Check sheet for the modelled part. Datum: model origin and axes. Units: mm. Face numbers are marked on the shaded views. A direction names the side the tool comes from. Give positions to 0.01 mm unless a question says otherwise; leave off trailing zeros. Loops run counter-clockwise (first coordinate to the right, second up) from the corner with the lowest first, then second, coordinate; pieces in that order, holes last. Notation, with made-up numbers: (41, 18.25) - (54, 18.25) arc R21 cw to (54, 40.25) - close; hole circle Ø5 at (38.5, -6). An arc over 180 degrees is marked (long way). Answer in a Markdown table with one row per item. Add a question column.
(1) Sectioned sample at B-B on z = 6. Enter the section's corners in (x, y).
(2) Sectioned sample at C-C on y = 1. Enter the section's corners in (x, z).
(3) Thickness scan on L1, parallel to Z at x = 53, y = 2; L2, parallel to Y at x = 39.5, z = 3.5. Record the ranges inside material, lowest first.
(4) Go/stop test with flat-tipped pins: P1, Ø6.5, axis at x = 59, z = 4.5, coming from the -Y side; P2, Ø1, axis at x = 37, y = 6.5, coming from the -Z side; P3, Ø9, axis at x = 21, z = 2, coming from the +Y side. Record where each tip stops, or that it passes through.
(5) Set-up check for the marked faces 1, 2 and 3: record each of +Z, -Z, +X, -X, +Y, -Y from which the full face is reachable in a straight line by a thin tool's end or side.
(6) Sectioned sample at A-A on x = 60.5. Enter the section's corners in (y, z).
from build123d import *

# Parameters (mm, degrees)
SKETCH1_W           = 80
SKETCH1_H           = 8.1
BOSS_EXTRUDE1_DEPTH = 20
CUT_EXTRUDE1_DEPTH  = 85


with BuildPart() as part:
    # Sketch1 → Boss-Extrude1 (new body)
    with BuildSketch(Plane.XY):
        with Locations((40, 4.05)):
            Rectangle(SKETCH1_W, SKETCH1_H)
    extrude(amount=BOSS_EXTRUDE1_DEPTH)

    # Sketch2 → Cut-Extrude1 (cut)
    with BuildSketch(Plane.ZY):
        Polygon((0, 8.1), (8, 8.1), (8, 5.9), (1.006469224, 5.9), (0, 5.9), align=None)
        Polygon((0, 0), (8, 0), (8, 2.2), (1.006469224, 2.2), (0, 2.2), align=None)
    extrude(amount=-CUT_EXTRUDE1_DEPTH, mode=Mode.SUBTRACT)


solid = part.part
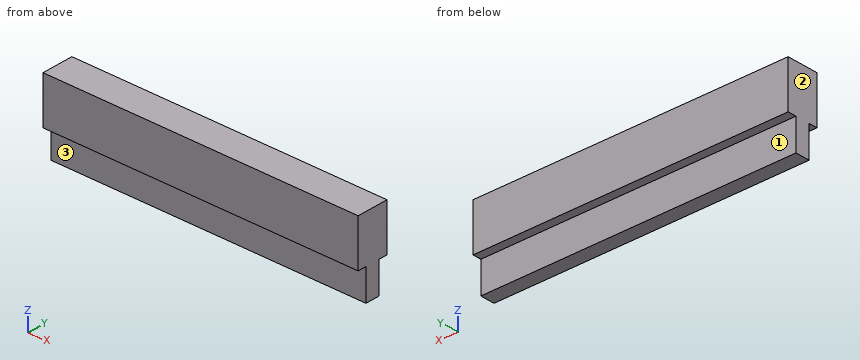
Reply:
| question | item | result |
|---|---|---|
| 1 | outline | (0, 2.2) - (80, 2.2) - (80, 5.9) - (0, 5.9) - close |
| 2 | outline | (0, 8) - (80, 8) - (80, 20) - (0, 20) - close |
| 3 | L1 | 8 to 20 |
| 3 | L2 | 2.2 to 5.9 |
| 4 | P1 | y = 2.2 |
| 4 | P2 | z = 8 |
| 4 | P3 | y = 5.9 |
| 5 | face 1 | -Z, +X, -X, +Y |
| 5 | face 2 | +Z, -Z, -X, +Y, -Y |
| 5 | face 3 | -Z, +X, -X, -Y |
| 6 | outline | (0, 8) - (2.2, 8) - (2.2, 0) - (5.9, 0) - (5.9, 8) - (8.1, 8) - (8.1, 20) - (0, 20) - close |
